```python
from build123d import *

# Parameters (mm, degrees)
F0_R     = 13.102935
F1_DEPTH = 6.35


with BuildPart() as f1:
    # F0 (on Top) → F1 (new body)
    with BuildSketch(Plane.XY):
        with BuildLine():
            Line((-65.111071, 33.079109), (-73.495406, 32.406889))
            ThreePointArc((-73.495406, 32.406889), (-102.707914, 0.699242), (-73.377358, -30.899239))
            Line((-73.377358, -30.899239), (-64.859611, -31.550194))
            ThreePointArc((-64.859611, -31.550194), (-53.305524, -34.288957), (-43.155709, -40.451666))
            Line((-43.155709, -40.451666), (-41.011948, -42.265209))
            ThreePointArc((-41.011948, -42.265209), (0, -57.285625), (41.011948, -42.265209))
            Line((41.011948, -42.265209), (43.152891, -40.45405))
            ThreePointArc((43.152891, -40.45405), (53.305798, -34.290073), (64.863456, -31.55207))
            Line((64.863456, -31.55207), (73.420082, -30.899652))
            ThreePointArc((73.420082, -30.899652), (102.756191, 0.699387), (73.537863, 32.407366))
            Line((73.537863, 32.407366), (65.115129, 33.081106))
            ThreePointArc((65.115129, 33.081106), (53.354307, 35.951298), (43.087573, 42.366053))
            Line((43.087573, 42.366053), (41.775827, 43.511932))
            ThreePointArc((41.775827, 43.511932), (0, 59.189026), (-41.775827, 43.511932))
            Line((-41.775827, 43.511932), (-43.090499, 42.363497))
            ThreePointArc((-43.090499, 42.363497), (-53.354005, 35.950102), (-65.111071, 33.079109))
        make_face()
        with Locations((-76.359481, 0)):
            Circle(F0_R, mode=Mode.SUBTRACT)
        with BuildLine():
            ThreePointArc((-44.465763, 0), (0, 44.465763), (44.465763, 0))
            ThreePointArc((44.465763, 0), (0, -44.465763), (-44.465763, 0))
        make_face(mode=Mode.SUBTRACT)
        with BuildLine():
            ThreePointArc((89.462416, 0), (76.359481, -13.102935), (63.256546, 0))
            ThreePointArc((63.256546, 0), (76.359481, 13.102935), (89.462416, 0))
        make_face(mode=Mode.SUBTRACT)
    extrude(amount=F1_DEPTH)


solid = f1.part
```
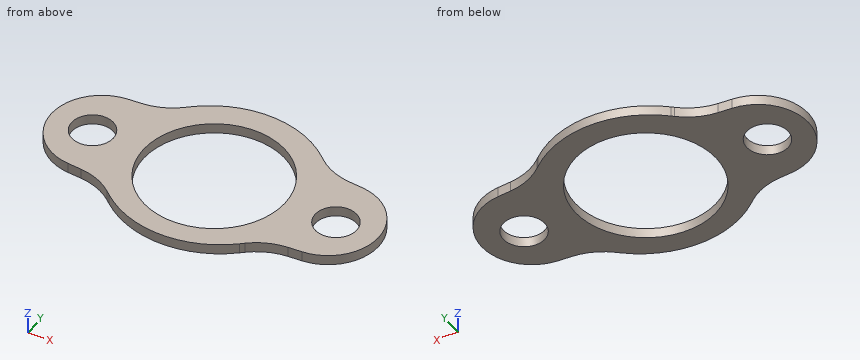
CAD build for the part. Positions are in the model's coordinates, mm. Give positions to 0.01 mm unless a question says otherwise; leave off trailing zeros. Order: outer loops, then holes, each group sorted by start corner. A loop starts at its lowest first (then second) coordinate and runs counter-clockwise, first axis right, second up.
(1) Saw through at D-D, the plane y = -37.5. Give the cut face in (x, z).
(2) Saw through at A-A, the plane x = 0. Give the cut face in (y, z).
(3) Flat gauge pins, fed straight in: pin 1 (3 mm diameter, centred on y = 21, z = 4.5, fed in from +X); pin 2 (1.5 mm diameter, centred on y = 47.5, z = 5.5, fed in from -X); pin 3 (23.5 mm diameter, centred on x = -76.36, y = 0, fed in from +Z) (3 decimals); pin 4 (1 mm diameter, centred on x = 65, z = 2, fed in from +Y). Where does each tip first touch, or does it go through?
(4) Drill centre lines: L1, parallel to X at y = -28.5, z = 1.25; L2, parallel to Y at x = 82.5, z = 4.75; L3, parallel to X at y = -41, z = 5.5. Where is each one in solid material? Low to high.
(5) Saw through at C-C, the plane z = 2.75. Give the cut face in (x, y), then the cut area to 3 significant figures.
(6) Saw through at B-B, the plane y = 0. Give the cut face in (x, z).
Results found:
1. outline: (-47.15, 0) - (-23.89, 0) - (-23.89, 6.35) - (-47.15, 6.35) - close; (23.89, 0) - (47.15, 0) - (47.15, 6.35) - (23.89, 6.35) - close
2. outline: (-57.29, 0) - (-44.47, 0) - (-44.47, 6.35) - (-57.29, 6.35) - close; (44.47, 0) - (59.19, 0) - (59.19, 6.35) - (44.47, 6.35) - close
3. pin 1: stops at x = 96.63
3. pin 2: stops at x = -37.75
3. pin 3: passes through
3. pin 4: stops at y = 33.14
4. L1: x = -83.29 to -34.13, 34.13 to 83.34
4. L2: y = -28.84 to -11.58, 11.58 to 30.36
4. L3: x = -42.51 to -17.21, 17.21 to 42.51
5. outline: (-73.5, 32.41) arc R31.75 ccw to (-73.38, -30.9) - (-64.86, -31.55) arc R38.1 cw to (-43.16, -40.45) - (-41.01, -42.27) arc R63.5 ccw to (41.01, -42.27) - (43.15, -40.45) arc R38.1 cw to (64.86, -31.55) - (73.42, -30.9) arc R31.75 ccw to (73.54, 32.41) - (65.12, 33.08) arc R38.1 cw to (43.09, 42.37) - (41.78, 43.51) arc R63.5 ccw to (-41.78, 43.51) - (-43.09, 42.36) arc R38.1 cw to (-65.11, 33.08) - close; hole circle Ø26.21 at (-76.36, 0); hole circle Ø88.93 at (0, 0); hole circle Ø26.21 at (76.36, 0)
5. area: 8,880 mm2
6. outline: (-102.7, 0) - (-89.46, 0) - (-89.46, 6.35) - (-102.7, 6.35) - close; (-63.26, 0) - (-44.47, 0) - (-44.47, 6.35) - (-63.26, 6.35) - close; (44.47, 0) - (63.26, 0) - (63.26, 6.35) - (44.47, 6.35) - close; (89.46, 0) - (102.75, 0) - (102.75, 6.35) - (89.46, 6.35) - close
